```python
from build123d import *

# Parameters (mm, degrees)
SKETCH1_R           = 30
SKETCH1_R_2         = 15
BOSS_EXTRUDE1_DEPTH = 10
SKETCH2_R           = 1.7
CUT_EXTRUDE1_DEPTH  = 44.588989435
CUT_EXTRUDE2_DEPTH  = 3
CIRPATTERN1_COUNT   = 4


with BuildPart() as part:
    # Sketch1 → Boss-Extrude1 (new body)
    with BuildSketch(Plane(origin=(0, 0, 0), x_dir=(1, 0, 0), z_dir=(0, 1, 0))):
        with Locations(Location((0, 0, 0), (0, 0, 270))):
            Circle(SKETCH1_R)
        with Locations(Location((0, 0, 0), (0, 0, 270))):
            Circle(SKETCH1_R_2, mode=Mode.SUBTRACT)
    extrude(amount=BOSS_EXTRUDE1_DEPTH)

    # Sketch2 → Cut-Extrude1 (cut, through all)
    with BuildSketch(Plane(origin=(0, 10, 0), x_dir=(1, 0, 0), z_dir=(0, 1, 0))):
        with Locations(Location((0, -20, 0), (0, 0, 270))):
            Circle(SKETCH2_R)
    cut_extrude1 = extrude(amount=-CUT_EXTRUDE1_DEPTH, mode=Mode.SUBTRACT)

    # Sketch3 → Cut-Extrude2 (cut)
    with BuildSketch(Plane.XZ):
        Polygon((3.464101615, 20), (1.732050808, 23), (-1.732050808, 23), (-3.464101615, 20), (-1.732050808, 17), (1.732050808, 17), align=None)
    cut_extrude2 = extrude(amount=-CUT_EXTRUDE2_DEPTH, mode=Mode.SUBTRACT)

    # CirPattern1: Cut-Extrude1, Cut-Extrude2 ×4 about axis
    cirpattern1_axis = Axis((0, 0, 0), (0, 1, 0))
    add([cut_extrude1.rotate(cirpattern1_axis, i * 360 / CIRPATTERN1_COUNT) for i in range(1, CIRPATTERN1_COUNT)], mode=Mode.SUBTRACT)
    add([cut_extrude2.rotate(cirpattern1_axis, i * 360 / CIRPATTERN1_COUNT) for i in range(1, CIRPATTERN1_COUNT)], mode=Mode.SUBTRACT)


solid = part.part
```
Here's how the part is built. I have some questions about the finished solid (model axes, mm). A direction names the side the tool comes from. Round coordinates to 2 decimals unless told otherwise and drop trailing zeros. Order: outer loops, then holes, each group sorted by start corner. A loop starts at its lowest first (then second) coordinate and runs counter-clockwise, first axis right, second up. Notation, with made-up numbers: M 72,-10 L 86,-10 A13 cw 86,4 Z; hole C 31.5,44.25 d3. An arc over 180 degrees is marked long. Answer in a Markdown table with one row per item.
Item 1: Imagine slicing it at D-D, the plane x = -8.5. Write out the boundary of the cut face in (y, z).
A:
| item | result |
|---|---|
| outline | M 0,-28.77 L 10,-28.77 L 10,-12.36 L 0,-12.36 Z; M 0,12.36 L 10,12.36 L 10,28.77 L 0,28.77 Z |
Item 2: Imagine slicing it at B-B, the plane y = 3.75. Write out the boundary of the cut face in (x, z), and give its area (3 significant figures).
A:
| item | result |
|---|---|
| outline | C 0,0 d60; hole C -20,0 d3.4; hole C 0,0 d30; hole C 0,-20 d3.4; hole C 0,20 d3.4; hole C 20,0 d3.4 |
| area | 2,080 mm2 |
Item 3: I'm going to push flat-ended pins straight in: pin 1 (3.5 mm diameter, centred on y = 1.5, z = -0.5, fed in from +X); pin 2 (2 mm diameter, centred on y = 1, z = 7, fed in from -X); pin 3 (2.5 mm diameter, centred on y = 1, z = 0, fed in from -X). Where does each tip first touch, or does it pass through?
A:
| item | result |
|---|---|
| pin 1 | stops at x = 30 |
| pin 2 | stops at x = -29.39 |
| pin 3 | stops at x = -30 |
Item 4: Imagine slicing it at A-A, the plane x = 0. Write out the boundary of the cut face in (y, z), and give its area (3 significant figures).
A:
| item | result |
|---|---|
| outline | M 0,-30 L 10,-30 L 10,-21.7 L 3,-21.7 L 3,-23 L 0,-23 Z; M 0,-17 L 3,-17 L 3,-18.3 L 10,-18.3 L 10,-15 L 0,-15 Z; M 0,15 L 10,15 L 10,18.3 L 3,18.3 L 3,17 L 0,17 Z; M 0,23 L 3,23 L 3,21.7 L 10,21.7 L 10,30 L 0,30 Z |
| area | 216 mm2 |
Item 5: Imagine slicing it at C-C, the plane z = -7. Write out the boundary of the cut face in (x, y).
A:
| item | result |
|---|---|
| outline | M -29.17,0 L -13.27,0 L -13.27,10 L -29.17,10 Z; M 13.27,0 L 29.17,0 L 29.17,10 L 13.27,10 Z |
Item 6: If I drill on L1, parallel to X at y = 2.5, z = 0; L2, parallel to Z at x = 1.5, y = 4; L3, parallel to X at y = 6.5, z = 18.5, over which ranges is the centre line in solid material (lowest first)? Write a range as from..to.
A:
| item | result |
|---|---|
| L1 | x = -30..-23, -17..-15, 15..17, 23..30 |
| L2 | z = -29.96..-20.8, -19.2..-14.92, 14.92..19.2, 20.8..29.96 |
| L3 | x = -23.62..-0.8, 0.8..23.62 |
Item 7: Thinking about a two-plate mould opening in X: for faces 3 (the face through (-18.5, 1.5, 2.6)), 4 (the face through (1.32, 4.93, -29.97)), 5 (the face through (14, 0, 6)), which applies, +X half, -X half, draft (parallel to the pull), parting line (faces both ways), or undercut?
A:
| item | result |
|---|---|
| face 3 | undercut |
| face 4 | parting line |
| face 5 | draft |
Item 8: For faces 1 (the face through (0, 1, -23)), 2 (the face through (21.57, 6.55, 0.65)), which set-ups out of +Z, -Z, +X, -X, +Y, -Y let a thin tool reach every point of the face, with its end or its side?
A:
| item | result |
|---|---|
| face 1 | -Y |
| face 2 | +Y, -Y |
